Read the model definition and answer for the solid it produces. Units are mm, in the model's axes. Face numbers are marked on the shaded views. A direction names the side the tool comes from. Coordinates: 2 decimals unless noted, no trailing zeros. Order: outer loops, then holes, each group sorted by start corner. A loop starts at its lowest first (then second) coordinate and runs counter-clockwise, first axis right, second up. Notation, with made-up numbers: (30, -30) -> (71, -30) arc R23 ccw to (71, -21) -> close; hole circle Ø2 at (74, 17). An arc over 180 degrees is marked (long way). Answer in a Markdown table with one row per item.
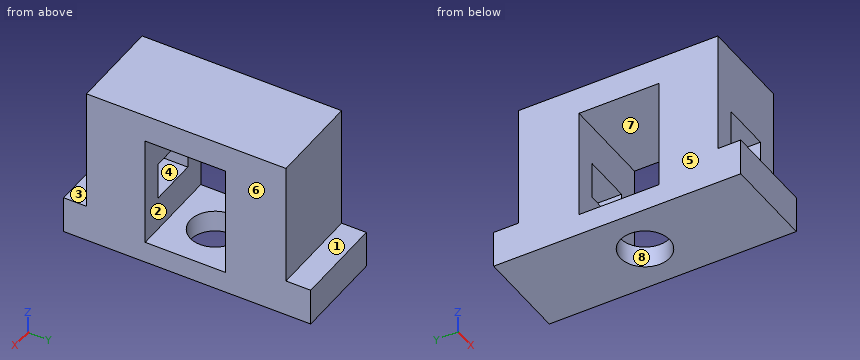
from build123d import *

# Parameters (mm, degrees)
F0_W     = 30
F0_H     = 80
F1_DEPTH = 52
F2_W     = 30
F2_H     = 8
F2_H_2   = 7.3947347701
F3_DEPTH = 40
F4_W     = 16
F4_H     = 12
F5_DEPTH = 64
F6_W     = 26
F6_H     = 36
F7_DEPTH = 30
F8_R     = 8
F9_DEPTH = 9


with BuildPart() as f1:
    # F0 (on Top) → F1 (new body)
    with BuildSketch(Plane.XY):
        with Locations((15, 40)):
            Rectangle(F0_W, F0_H)
    extrude(amount=F1_DEPTH)

    # F2 (on face) → F3 (cut)
    with BuildSketch(Plane.XY.offset(52)):
        with Locations((15, 76)):
            Rectangle(F2_W, F2_H)
        with Locations((15, 3.697367385)):
            Rectangle(F2_W, F2_H_2)
    extrude(amount=-F3_DEPTH, mode=Mode.SUBTRACT)

    # F4 (on face) → F5 (cut)
    with BuildSketch(Plane.XZ.offset(-7.3947347701)):
        with Locations((15, 24)):
            Rectangle(F4_W, F4_H)
    extrude(amount=-F5_DEPTH, mode=Mode.SUBTRACT)

    # F6 (on face) → F7 (cut)
    with BuildSketch(Plane.YZ.offset(30)):
        with Locations((39.3947347701, 25)):
            Rectangle(F6_W, F6_H)
    extrude(amount=-F7_DEPTH, mode=Mode.SUBTRACT)

    # F8 (on face) → F9 (cut)
    with BuildSketch(Plane(origin=(0, 0, 0), x_dir=(1, 0, 0), z_dir=(0, 0, -1))):
        with Locations((15, -40)):
            Circle(F8_R)
    extrude(amount=-F9_DEPTH, mode=Mode.SUBTRACT)


solid = f1.part
Q1. For the marked faces 1, 2, 3 and 4, determine the directions among +Z, -Z, +X, -X, +Y, -Y from which every point of the face is accessible in a straight line to the end or side of a thin tool.
Outcome:
| item | result |
|---|---|
| face 1 | +Z, +X, -X, +Y |
| face 2 | +X, -X |
| face 3 | +Z, +X, -X, -Y |
| face 4 | -Y |
Q2. Given pin 1 (12 mm diameter, centred on x = 25, z = 42, fed in from -Y); pin 2 (6 mm diameter, centred on x = 12.5, z = 16.5, fed in from +Y); pin 3 (4 mm diameter, centred on x = 20, y = 78, fed in from +Z), each flat-ended and moving along its own axis, determine where each tip first touches the part or whether it passes through.
Outcome:
| item | result |
|---|---|
| pin 1 | y = 7.39 |
| pin 2 | y = 72 |
| pin 3 | z = 12 |
Q3. The part is cut by section D-D (y = 40). Write down the section's boundary in (x, z).
Outcome:
| item | result |
|---|---|
| outline | (0, 0) -> (7, 0) -> (7, 7) -> (0, 7) -> close; (0, 43) -> (30, 43) -> (30, 52) -> (0, 52) -> close; (23, 0) -> (30, 0) -> (30, 7) -> (23, 7) -> close |
Q4. The part is cut by section A-A (z = 33). Write down the section's boundary in (x, y).
Outcome:
| item | result |
|---|---|
| outline | (0, 7.39) -> (30, 7.39) -> (30, 26.39) -> (0, 26.39) -> close; (0, 52.39) -> (30, 52.39) -> (30, 72) -> (0, 72) -> close |
Q5. Consider line 1 (Y direction, x = 15, z = 4.25); line 2 (Y direction, x = 9.5, z = 15); line 3 (Z direction, x = 8, y = 58). Determine where each line is inside the solid, lowest interval first.
Outcome:
| item | result |
|---|---|
| line 1 | 0 to 32, 48 to 80 |
| line 2 | 7.39 to 26.39, 52.39 to 72 |
| line 3 | 0 to 18, 30 to 52 |
Q6. The part is cut by section C-C (x = 15). Write down the section's boundary in (y, z).
Outcome:
| item | result |
|---|---|
| outline | (0, 0) -> (32, 0) -> (32, 7) -> (26.39, 7) -> (26.39, 18) -> (7.39, 18) -> (7.39, 12) -> (0, 12) -> close; (7.39, 30) -> (26.39, 30) -> (26.39, 43) -> (52.39, 43) -> (52.39, 30) -> (71.39, 30) -> (71.39, 18) -> (52.39, 18) -> (52.39, 7) -> (48, 7) -> (48, 0) -> (80, 0) -> (80, 12) -> (72, 12) -> (72, 52) -> (7.39, 52) -> close |
Q7. The part is cut by section B-B (y = 63). Write down the section's boundary in (x, z).
Outcome:
| item | result |
|---|---|
| outline | (0, 0) -> (30, 0) -> (30, 52) -> (0, 52) -> close; hole (7, 18) -> (23, 18) -> (23, 30) -> (7, 30) -> close |
Q8. For a pull along X with two mould halves and no side action, classify the marked faces 5, 6, 7 and 8 as pulls with the +X half, pulls with the -X half, needs draft (parallel to the pull), parting line crosses it, or undercut.
Outcome:
| item | result |
|---|---|
| face 5 | pulls with the -X half |
| face 6 | pulls with the +X half |
| face 7 | needs draft |
| face 8 | undercut |
